Source: CAD feature listing. Evaluate the final solid. Frame: model axes, mm. A direction names the side the tool comes from. Coordinates: 2 decimals unless noted, no trailing zeros. Write each loop counter-clockwise with the first axis right and the second up, starting at its lowest first coordinate (ties: lowest second). Pieces come first, ordered by that corner, then holes. Notation, with made-up numbers: (-16, 72) - (26, 72) arc R20 ccw to (26, 97) - close; hole circle Ø4 at (29, -12.75). An arc over 180 degrees is marked (long way). One line per item, written item: value.
from build123d import *

# Parameters (mm, degrees)
F1_DEPTH  = 7
F3_DEPTH  = 26
F4_R      = 2.45
F5_DEPTH  = 7
F6_R      = 2
F7_R      = 1.5
F8_DEPTH  = 77.001
F9_R      = 4
F10_DEPTH = 70
F11_R     = 1.55
F12_DEPTH = 26.001
F13_W     = 58
F13_H     = 6
F14_DEPTH = 10


with BuildPart() as f1:
    # F0 (on Top) → F1 (new body)
    with BuildSketch(Plane.XY):
        with BuildLine():
            Line((0, 45), (0, 0))
            Line((0, 0), (5.660254, 0))
            ThreePointArc((5.660254, 0), (6.954349, 0.170371), (8.160254, 0.669873))
            Line((8.160254, 0.669873), (21.428203, 8.330127))
            ThreePointArc((21.428203, 8.330127), (22.634108, 8.829629), (23.928203, 9))
            Line((23.928203, 9), (72, 9))
            ThreePointArc((72, 9), (75.535534, 10.464466), (77, 14))
            Line((77, 14), (77, 31.6017))
            ThreePointArc((77, 31.6017), (75.754201, 34.90412), (72.637609, 36.560879))
            Line((72.637609, 36.560879), (7, 45))
            Line((7, 45), (0, 45))
        make_face()
    extrude(amount=F1_DEPTH)

    # F2 (on face) → F3 (join)
    with BuildSketch(Plane.XY.offset(7)):
        with BuildLine():
            Line((0, 45), (0, 0))
            Line((0, 0), (7, 0))
            Line((7, 0), (7, 19))
            Line((7, 19), (77, 19))
            Line((77, 19), (77, 31.6017))
            ThreePointArc((77, 31.6017), (75.754201, 34.90412), (72.637609, 36.560879))
            Line((72.637609, 36.560879), (7, 45))
            Line((7, 45), (0, 45))
        make_face()
    extrude(amount=F3_DEPTH)

    # F4 (on face) → F5 (join)
    with BuildSketch(Plane.XY.offset(33)):
        with BuildLine():
            Line((0, 45), (0, 0))
            Line((0, 0), (5.660254, 0))
            ThreePointArc((5.660254, 0), (6.954349, 0.170371), (8.160254, 0.669873))
            Line((8.160254, 0.669873), (21.483041, 8.361788))
            ThreePointArc((21.483041, 8.361788), (22.688946, 8.86129), (23.983041, 9.03166))
            Line((23.983041, 9.03166), (72, 9.03166))
            ThreePointArc((72, 9.03166), (75.535534, 10.496127), (77, 14.03166))
            Line((77, 14.03166), (77, 31.631387))
            ThreePointArc((77, 31.631387), (75.753466, 34.934642), (72.635402, 36.590849))
            Line((72.635402, 36.590849), (7, 45))
            Line((7, 45), (0, 45))
        make_face()
        with BuildLine():
            Line((-23, 0), (0, 0))
            Line((0, 0), (0, 45))
            Line((0, 45), (-23, 45))
            ThreePointArc((-23, 45), (-26.535534, 43.535534), (-28, 40))
            Line((-28, 40), (-28, 5))
            ThreePointArc((-28, 5), (-26.535534, 1.464466), (-23, 0))
        make_face()
        with Locations((-7, 16.5)):
            Circle(F4_R, mode=Mode.SUBTRACT)
        with Locations((-23, 27.5)):
            Circle(F4_R, mode=Mode.SUBTRACT)
    extrude(amount=F5_DEPTH)

    # F6
    f6_edges = [f1.edges().sort_by_distance(p)[0] for p in [
        (-9.45, 16.5, 33),
        (-25.45, 27.5, 33),
    ]]
    fillet(f6_edges, radius=F6_R)

    # F7 (on face) → F8 (cut, through all)
    with BuildSketch(Plane(origin=(0, 0, 0), x_dir=(0, -1, 0), z_dir=(-1, 0, 0))):
        with Locations((-32.5, 30)):
            Circle(F7_R)
        with Locations((-12.5, 30)):
            Circle(F7_R)
        with Locations((-12.5, 10)):
            Circle(F7_R)
        with Locations((-32.5, 10)):
            Circle(F7_R)
    extrude(amount=-F8_DEPTH, mode=Mode.SUBTRACT)

    # F9 (on face) → F10 (cut)
    with BuildSketch(Plane.YZ.offset(77)):
        with Locations((32.5, 30)):
            Circle(F9_R)
        with Locations((32.5, 10)):
            Circle(F9_R)
    extrude(amount=-F10_DEPTH, mode=Mode.SUBTRACT)

    # F11 (on face) → F12 (cut, through all)
    with BuildSketch(Plane.XZ.offset(-19)):
        with Locations((22, 20)):
            Circle(F11_R)
        with Locations((47, 20)):
            Circle(F11_R)
        with Locations((72, 20)):
            Circle(F11_R)
    extrude(amount=-F12_DEPTH, mode=Mode.SUBTRACT)

    # F13 (on face) → F14 (cut)
    with BuildSketch(Plane(origin=(0, 45, 0), x_dir=(-1, 0, 0), z_dir=(0, 1, 0))):
        with Locations((-46, 20)):
            Rectangle(F13_W, F13_H)
    extrude(amount=-F14_DEPTH, mode=Mode.SUBTRACT)


solid = f1.part
1) Section query B-B on z = 20. Output: boundary loops of the cut face in (x, y).
Values found:
outline: (0, 0) - (7, 0) - (7, 19) - (20.45, 19) - (20.45, 35) - (17, 35) - (17, 43.71) - (7, 45) - (0, 45) - close; (23.55, 19) - (45.45, 19) - (45.45, 35) - (23.55, 35) - close; (48.55, 19) - (70.45, 19) - (70.45, 35) - (48.55, 35) - close; (73.55, 19) - (77, 19) - (77, 31.6) arc R5 ccw to (75, 35.6) - (75, 35) - (73.55, 35) - close
2) Reachability of faces 1 (the flat face through (40, 38, 17)), 2 (the cylindrical face through (42.49, 31.979, 33.966)), 3 (the cylindrical face through (6.937, 0.166, 3.451)) from +Z, -Z, +X, -X, +Y, -Y: full face, straight path, thin tool, end or side. Return the list, or none.
Values found:
face 1: +Y
face 2: +X
face 3: -Z, +X, -Y
3) Material intervals for line 1 (Z direction, x = 20.5, y = 13.5); line 2 (Z direction, x = 22, y = 31); line 3 (Y direction, x = -7, z = 37), sorted ascending.
Values found:
line 1: 0 to 7, 33 to 40
line 2: 0 to 6.29, 13.71 to 18.45, 21.55 to 26.29, 33.71 to 40
line 3: 0 to 14.05, 18.95 to 45
4) Contact query for flat-ended pins moving along their axis: P1, Ø1.5, axis at y = 14.5, z = 7, coming from the -X side; P2, Ø2, axis at y = 11.5, z = 4.5, coming from the +X side; P3, Ø3, axis at y = 34, z = 31, coming from the +X side; P4, Ø1, axis at x = 45, y = 18, coming from the -Z side. Output: stop coordinate, or through.
Values found:
P1: x = 0
P2: x = 76.77
P3: x = 7
P4: z = 0
5) Section query A-A on y = 27.5. Output: boundary loops of the cut face in (x, z), then the cut area to 3 significant figures.
Values found:
outline: (-28, 33) - (-27.45, 33) arc R2 ccw to (-25.45, 35) - (-25.45, 40) - (-28, 40) - close; (-20.55, 35) arc R2 ccw to (-18.55, 33) - (0, 33) - (0, 0) - (77, 0) - (77, 40) - (-20.55, 40) - close; hole circle Ø3.1 at (22, 20); hole circle Ø3.1 at (47, 20); hole circle Ø3.1 at (72, 20)
area: 3,220 mm2
6) Section query D-D on y = 16.5. Output: boundary loops of the cut face in (x, z).
Values found:
outline: (-28, 33) - (-11.45, 33) arc R2 ccw to (-9.45, 35) - (-9.45, 40) - (-28, 40) - close; (-4.55, 35) arc R2 ccw to (-2.55, 33) - (0, 33) - (0, 0) - (77, 0) - (77, 7) - (7, 7) - (7, 33) - (77, 33) - (77, 40) - (-4.55, 40) - close
7) Draft query along X for faces 4 (the cylindrical face through (-27, 2, 36)), 5 (the cylindrical face through (48.478, 26.888, 20.466)), 6 (the flat face through (2, 45, 29)), 7 (the cylindrical face through (75.787, 34.866, 16.269)). Return one class per face: released by +X, released by -X, zero draft, split by the parting line, or undercut.
Values found:
face 4: released by -X
face 5: undercut
face 6: zero draft
face 7: released by +X
8) Section query C-C on x = -7. Output: boundary loops of the cut face in (y, z).
Values found:
outline: (0, 33) - (12.05, 33) arc R2 ccw to (14.05, 35) - (14.05, 40) - (0, 40) - close; (18.95, 35) arc R2 ccw to (20.95, 33) - (45, 33) - (45, 40) - (18.95, 40) - close
